from build123d import *

# Parameters (mm, degrees)
BOSS_EXTRUDE1_DEPTH = 60.96
CUT_EXTRUDE1_DEPTH  = 101.6
CUT_EXTRUDE2_DEPTH  = 7.62
SKETCH6_R           = 12.065
CUT_EXTRUDE3_DEPTH  = 12.7
SKETCH7_R           = 3.81
CUT_EXTRUDE5_DEPTH  = 102.631745151


with BuildPart() as part:
    # Sketch3 → Boss-Extrude1 (new body)
    with BuildSketch(Plane.XY):
        with BuildLine():
            Line((-27.94, 0.030892605), (27.94, 0.030892605))
            ThreePointArc((27.94, 0.030892605), (36.920256121, -3.688851274), (40.64, -12.669107395))
            Line((40.64, -12.669107395), (40.64, -43.149107395))
            Line((40.64, -43.149107395), (50.8, -43.149107395))
            Line((50.8, -43.149107395), (50.8, -6.319107395))
            ThreePointArc((50.8, -6.319107395), (48.812332806, 3.530901366), (43.160419482, 11.83929286))
            ThreePointArc((43.160419482, 11.83929286), (40.447471444, 15.733062174), (39.353319429, 20.350892605))
            Line((39.353319429, 20.350892605), (13.318319429, 20.350892605))
            Line((13.318319429, 20.350892605), (13.318319429, 16.540892605))
            Line((13.318319429, 16.540892605), (-10.811680571, 16.540892605))
            Line((-10.811680571, 16.540892605), (-10.811680571, 20.350892605))
            Line((-10.811680571, 20.350892605), (-36.846680571, 20.350892605))
            ThreePointArc((-36.846680571, 20.350892605), (-37.999423394, 15.718716246), (-40.780780624, 11.83929286))
            ThreePointArc((-40.780780624, 11.83929286), (-47.728103025, 3.829260087), (-50.8, -6.319107395))
            Line((-50.8, -6.319107395), (-50.8, -43.149107395))
            Line((-50.8, -43.149107395), (-40.64, -43.149107395))
            Line((-40.64, -43.149107395), (-40.64, -12.669107395))
            ThreePointArc((-40.64, -12.669107395), (-36.920256121, -3.688851274), (-27.94, 0.030892605))
        make_face()
    extrude(amount=-BOSS_EXTRUDE1_DEPTH)

    # Sketch4 → Cut-Extrude1 (cut)
    with BuildSketch(Plane(origin=(50.8, 0, 0), x_dir=(0, 0, -1), z_dir=(1, 0, 0))):
        with BuildLine():
            Line((12.7, -43.149107395), (12.7, -23.591107395))
            ThreePointArc((12.7, -23.591107395), (30.48, -11.3802667), (48.26, -23.591107395))
            Line((48.26, -23.591107395), (48.26, -43.149107395))
            Line((48.26, -43.149107395), (12.7, -43.149107395))
        make_face()
    extrude(amount=-CUT_EXTRUDE1_DEPTH, mode=Mode.SUBTRACT)

    # Sketch5 → Cut-Extrude2 (cut)
    with BuildSketch(Plane(origin=(0, 20.350892605, 0), x_dir=(1, 0, 0), z_dir=(0, 1, 0))):
        with BuildLine():
            Line((-20.844680571, 45.212), (-20.844680571, 15.748))
            ThreePointArc((-20.844680571, 15.748), (-19.803152285, 13.233528286), (-17.288680571, 12.192))
            Line((-17.288680571, 12.192), (19.795319429, 12.192))
            ThreePointArc((19.795319429, 12.192), (22.309791143, 13.233528286), (23.351319429, 15.748))
            Line((23.351319429, 15.748), (23.351319429, 45.212))
            ThreePointArc((23.351319429, 45.212), (22.309791143, 47.726471714), (19.795319429, 48.768))
            Line((19.795319429, 48.768), (-17.288680571, 48.768))
            ThreePointArc((-17.288680571, 48.768), (-19.803152285, 47.726471714), (-20.844680571, 45.212))
        make_face()
    extrude(amount=-CUT_EXTRUDE2_DEPTH, mode=Mode.SUBTRACT)

    # Sketch6 → Cut-Extrude3 (cut)
    with BuildSketch(Plane(origin=(0, 12.730892605, 0), x_dir=(1, 0, 0), z_dir=(0, 1, 0))):
        with Locations(Location((0, 30.48, 0), (0, 0, 180))):
            Circle(SKETCH6_R)
    extrude(amount=-CUT_EXTRUDE3_DEPTH, mode=Mode.SUBTRACT)

    # Sketch7 → Cut-Extrude5 (cut, through all)
    with BuildSketch(Plane(origin=(0, 20.350892605, 0), x_dir=(1, 0, 0), z_dir=(0, 1, 0))):
        with Locations(Location((-29.226680571, 52.705, 0), (0, 0, 180))):
            Circle(SKETCH7_R)
        with Locations(Location((31.733319429, 52.705, 0), (0, 0, 180))):
            Circle(SKETCH7_R)
        with Locations(Location((31.733319429, 8.255, 0), (0, 0, 180))):
            Circle(SKETCH7_R)
        with Locations(Location((-29.226680571, 8.255, 0), (0, 0, 180))):
            Circle(SKETCH7_R)
    extrude(amount=-CUT_EXTRUDE5_DEPTH, mode=Mode.SUBTRACT)


solid = part.part
Model file for the job. Use its own axes, mm. A direction names the side the tool comes from. Give positions to 0.01 mm unless a question says otherwise; leave off trailing zeros. Order: outer loops, then holes, each group sorted by start corner. A loop starts at its lowest first (then second) coordinate and runs counter-clockwise, first axis right, second up. Notation, with made-up numbers: (12, 80.25) - (44, 80.25) arc R28 cw to (44, 107.25) - close; hole circle Ø1 at (-28.75, -22.5). An arc over 180 degrees is marked (long way). Write item = value, one per line. Start each with the question number.
1. Two-plate mould, pull along X, no slides. Class faces 1 (the flat face through (-27, 20.351, -30)), 2 (the cylindrical face through (48.867, 3.4, -30.053)), 3 (the flat face through (1, 16, -12.192)), 4 (the cylindrical face through (22.282, 16.594, -13.206)): pulls with the +X half, pulls with the -X half, needs draft (parallel to the pull), parting line crosses it, or undercut.
2. Cut at A-A, the plane z = -30.48. List the corners of the cut face in (x, y) (1 decimal), and give its area (3 significant figures).
3. Cut at B-B, the plane x = 0. List the corners of the cut face in (y, z) (3 decimals), and give its area (3 significant figures).
4. Cut at D-D, the plane x = 17.5. List the corners of the cut face in (y, z).
5. Cut at C-C, the plane y = 4.5. List the corners of the cut face in (x, z) (3 decimals), and give its area (3 significant figures).
6. Drop flat-ended pins along their axis: P1, Ø4, axis at x = -5, y = 18.5, coming from the -Z side; P2, Ø2.5, axis at y = 18, z = -37.5, coming from the +X side; P3, Ø1.5, axis at x = 0.5, z = -45, coming from the -Y side; P4, Ø10, axis at x = 30, z = -26, coming from the -Y side. Give the stop position or say it passes through.
7. Which spindle directions (+Z, -Z, +X, -X, +Y, -Y) get a long thin tool onto all of the face, cutting with end or side? Do faces 5 (the flat face through (2, 16, -48.768)), 6 (the flat face through (1, 16.541, -6)), 7 (the flat face through (-46, -34, -12.7)), 8 (the cylindrical face through (-31.27, 9.81, -49.49)), 9 (the flat face through (40.64, -28, -6)). Say none if no direction does.
8. Probe line 1 along X through (y, z) = (-27, -50.5); line 2 along Z through (x, y) = (0, 8.25) (3 decimals); line 3 along Y through (x, z) = (23, -10). List the from-to ranges inside material, lowest first.
Taken from the geometry:
q1.face_1 = needs draft
q1.face_2 = pulls with the +X half
q1.face_3 = undercut
q1.face_4 = undercut
q2.outline = (-50.8, -11.4) - (-40.6, -11.4) arc R12.7 cw to (-27.9, 0) - (-12.1, 0) - (-12.1, 12.7) - (-20.8, 12.7) - (-20.8, 20.4) - (-36.8, 20.4) arc R12.7 cw to (-40.8, 11.8) arc R25.4 ccw to (-50.8, -6.3) - close; (12.1, 0) - (27.9, 0) arc R12.7 cw to (40.6, -11.4) - (50.8, -11.4) - (50.8, -6.3) arc R25.4 ccw to (43.2, 11.8) arc R12.7 cw to (39.4, 20.4) - (23.4, 20.4) - (23.4, 12.7) - (12.1, 12.7) - close
q2.area = 1,420 mm²
q3.outline = (0.031, -60.96) - (16.541, -60.96) - (16.541, -48.768) - (12.731, -48.768) - (12.731, -42.545) - (0.031, -42.545) - close; (0.031, -18.415) - (12.731, -18.415) - (12.731, -12.192) - (16.541, -12.192) - (16.541, 0) - (0.031, 0) - close
q3.area = 561 mm²
q4.outline = (0.03, -60.96) - (20.35, -60.96) - (20.35, -48.77) - (12.73, -48.77) - (12.73, -12.19) - (20.35, -12.19) - (20.35, 0) - (0.03, 0) - close
q5.outline = (-47.345, -60.96) - (48.381, -60.96) - (48.381, 0) - (-47.345, 0) - close; hole circle Ø7.62 at (-29.227, -52.705); hole circle Ø7.62 at (-29.227, -8.255); hole circle Ø24.13 at (0, -30.48); hole circle Ø7.62 at (31.733, -52.705); hole circle Ø7.62 at (31.733, -8.255)
q5.area = 5,200 mm²
q6.P1 = -60.96
q6.P2 = 40.04
q6.P3 = 0.03
q6.P4 = -2.11
q7.face_5 = +Y
q7.face_6 = +Z, -Z, +Y
q7.face_7 = +X, -X, -Y
q7.face_8 = +Y, -Y
q7.face_9 = +Z, -Z, -Y
q8.line_1 = -50.8 to -40.64, 40.64 to 50.8
q8.line_2 = -60.96 to -42.545, -18.415 to 0
q8.line_3 = 0.03 to 20.35
